Verification items for the finished model (mm, model axes). Face numbers are marked on the shaded views. Coordinates: 2 decimals unless noted, no trailing zeros. Order: outer loops, then holes, each group sorted by start corner. A loop starts at its lowest first (then second) coordinate and runs counter-clockwise, first axis right, second up.
Q1. Depth check by flat-ended pin: P1, Ø2.5, axis at x = -0.5, z = 2.5, coming from the +Y side; P2, Ø1.5, axis at x = -0.5, z = 9.5, coming from the +Y side (3 decimals); P3, Ø0.7, axis at x = 0, z = 2, coming from the -Y side; P4, Ø1.5, axis at x = -2, y = -1.5, coming from the -Z side. Enter the tip coordinate at first touch or a pass-through.
Q2. Cross-section at B-B, the plane z = 16. Record the boundary of the cut face in (x, y) (3 decimals), and give its area (3 significant figures).
Q3. Draft check along X on the marked faces 1, 2 and 3. Enter one of: pulls with the +X half, pulls with the -X half, needs draft (parallel to the pull), parting line crosses it, or undercut.
Q4. Cross-section at A-A, the plane x = 0. Record the boundary of the cut face in (y, z) (3 decimals).
Q5. Cross-section at C-C, the plane y = 0.5. Record the boundary of the cut face in (x, z).
Q6. Thickness scan on line 1 (X direction, y = -0.25, z = 35); line 2 (Z direction, x = 0, y = -0.25); line 3 (Z direction, x = 2.5, y = -0.75). Record the ranges inside material, lowest first.
from build123d import *

# Parameters (mm, degrees)
F0_W          = 3.175
F0_H          = 50.8
F2_R          = 4.7625
F3_DEPTH      = 4.826
F4_R          = 12.7
F5_DEPTH      = 3.176
F5_DEPTH_BACK = 3.176


with BuildPart() as f1:
    # F0 (on Front) → F1 (revolve)
    with BuildSketch(Plane.XZ):
        with Locations((1.5875, 25.4)):
            Rectangle(F0_W, F0_H)
    revolve(axis=Axis((0, 0, 31.9059565663), (0, 0, 1)))

    # F2 (on face) → F3 (cut)
    with BuildSketch(Plane(origin=(0, 0, 0), x_dir=(1, 0, 0), z_dir=(0, 0, -1))):
        Circle(F2_R)
        Polygon((-2.2913588808, 0), (-1.1456794404, 1.984375), (1.1456794404, 1.984375), (2.2913588808, 0), (1.1456794404, -1.984375), (-1.1456794404, -1.984375), align=None, mode=Mode.SUBTRACT)
    extrude(amount=-F3_DEPTH, mode=Mode.SUBTRACT)

    # F4 (on Front) → F5 (cut, two sides)
    with BuildSketch(Plane.XZ) as f5_sk:
        with Locations((0, -12.192)):
            Circle(F4_R)
    extrude(amount=-F5_DEPTH, mode=Mode.SUBTRACT)
    extrude(f5_sk.sketch, amount=F5_DEPTH_BACK, mode=Mode.SUBTRACT)


solid = f1.part
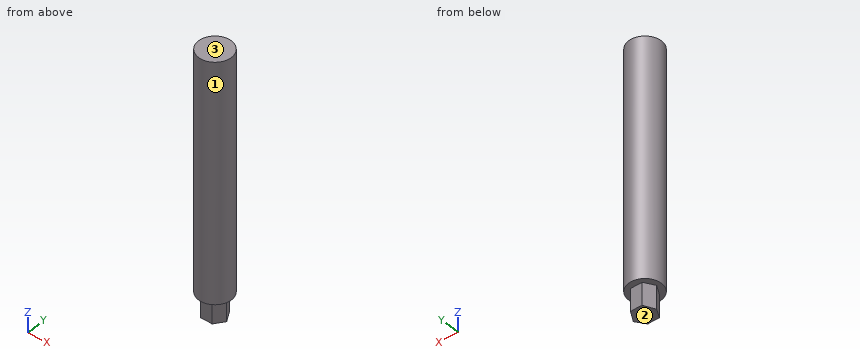
Check values:
1. P1: stops at y = 1.98
1. P2: stops at y = 3.175
1. P3: stops at y = -1.98
1. P4: stops at z = 0.37
2. outline: circle Ø6.35 at (0, 0)
2. area: 31.7 mm2
3. face 1: parting line crosses it
3. face 2: undercut
3. face 3: needs draft
4. outline: (-3.175, 4.826) - (-1.984, 4.826) - (-1.984, 0.508) - (1.984, 0.508) - (1.984, 4.826) - (3.175, 4.826) - (3.175, 50.8) - (-3.175, 50.8) - close
5. outline: (-3.14, 4.83) - (-2, 4.83) - (-2, 0.35) arc R12.7 cw to (2, 0.35) - (2, 4.83) - (3.14, 4.83) - (3.14, 50.8) - (-3.14, 50.8) - close
6. line 1: x = -3.17 to 3.17
6. line 2: z = 0.51 to 50.8
6. line 3: z = 4.83 to 50.8
